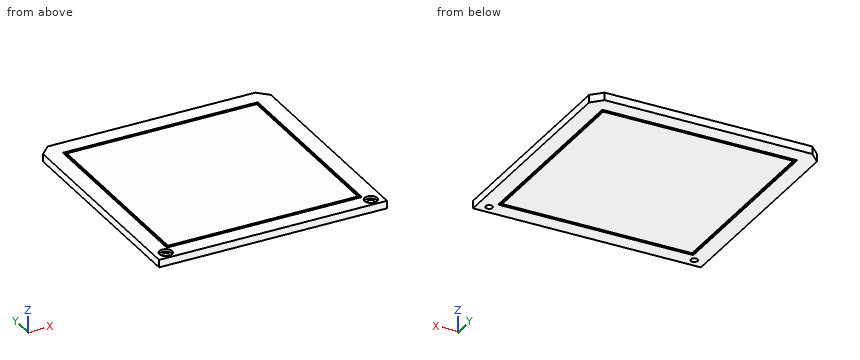
```python
from build123d import *

# Parameters (mm, degrees)
SKETCH1_W           = 90
SKETCH1_H           = 90
BOSS_EXTRUDE1_DEPTH = 3
SKETCH2_R           = 1.35
CUT_EXTRUDE1_DEPTH  = 4
SKETCH3_W           = 77
SKETCH3_H           = 77
SKETCH3_W_2         = 75
SKETCH3_H_2         = 75
CUT_EXTRUDE2_DEPTH  = 0.4
SKETCH4_W           = 77
SKETCH4_H           = 77
SKETCH4_W_2         = 75
SKETCH4_H_2         = 75
CUT_EXTRUDE3_DEPTH  = 0.4
CHAMFER1_SIZE       = 4
SKETCH5_R           = 2.5
CUT_EXTRUDE4_DEPTH  = 1


with BuildPart() as part:
    # Sketch1 → Boss-Extrude1 (new body)
    with BuildSketch(Plane.XY):
        Rectangle(SKETCH1_W, SKETCH1_H)
    extrude(amount=BOSS_EXTRUDE1_DEPTH)

    # Sketch2 → Cut-Extrude1 (cut, through all)
    with BuildSketch(Plane.XY.offset(3)):
        with Locations((-40.5, -41.5)):
            Circle(SKETCH2_R)
        with Locations((40.5, -41.5)):
            Circle(SKETCH2_R)
    extrude(amount=-CUT_EXTRUDE1_DEPTH, mode=Mode.SUBTRACT)

    # Sketch3 → Cut-Extrude2 (cut)
    with BuildSketch(Plane.XY.offset(3)):
        Rectangle(SKETCH3_W, SKETCH3_H)
        Rectangle(SKETCH3_W_2, SKETCH3_H_2, mode=Mode.SUBTRACT)
    extrude(amount=-CUT_EXTRUDE2_DEPTH, mode=Mode.SUBTRACT)

    # Sketch4 → Cut-Extrude3 (cut)
    with BuildSketch(Plane(origin=(0, 0, 0), x_dir=(-1, 0, 0), z_dir=(0, 0, -1))):
        Rectangle(SKETCH4_W, SKETCH4_H)
        Rectangle(SKETCH4_W_2, SKETCH4_H_2, mode=Mode.SUBTRACT)
    extrude(amount=-CUT_EXTRUDE3_DEPTH, mode=Mode.SUBTRACT)

    # Chamfer1
    chamfer1_edges = [part.edges().sort_by_distance(p)[0] for p in [
        (-45, 45, 1.5),
        (45, 45, 1.5),
    ]]
    chamfer(chamfer1_edges, length=CHAMFER1_SIZE)

    # Sketch5 → Cut-Extrude4 (cut)
    with BuildSketch(Plane.XY.offset(3)):
        with Locations((-40.5, -41.5)):
            Circle(SKETCH5_R)
        with Locations((40.5, -41.5)):
            Circle(SKETCH5_R)
    extrude(amount=-CUT_EXTRUDE4_DEPTH, mode=Mode.SUBTRACT)


solid = part.part
```
Work out the finished part from the listing and answer in its coordinate system (mm). Give positions to 0.01 mm unless a question says otherwise; leave off trailing zeros. Loops run counter-clockwise (first coordinate to the right, second up) from the corner with the lowest first, then second, coordinate; pieces in that order, holes last. Notation, with made-up numbers: (6.25, -16) - (28.25, -16) arc R6 ccw to (28.25, -6) - close; hole circle Ø1 at (8, 39.25). An arc over 180 degrees is marked (long way). Use CSV: the item, a comma, the result in double quotes. Start each with the question number.
(1) Find the intervals of material crossed by L1, parallel to X at y = 15.5, z = 2.9; L2, parallel to Y at x = 40.5, z = 1.4; L3, parallel to Y at x = -39.5, z = 1.2, in increasing order.
(2) This flat-tipped pin is pushed along its axis until it touches: pin 1 (8 mm diameter, centred on x = 26.5, y = 33.5, fed in from -Z). Where does it stop, or does it pass through?
(3) Find section A-A, the plane y = -41.5. Determine the outline of the cut face in (x, z), plus the area to 3 significant figures.
Results found:
1,L1,"-45 to -38.5, -37.5 to 37.5, 38.5 to 45"
1,L2,"-45 to -42.85, -40.15 to 45"
1,L3,"-45 to -42.41, -40.59 to 45"
2,pin 1,"z = 0"
3,outline,"(-45, 0) - (-41.85, 0) - (-41.85, 2) - (-43, 2) - (-43, 3) - (-45, 3) - close; (-39.15, 0) - (39.15, 0) - (39.15, 2) - (38, 2) - (38, 3) - (-38, 3) - (-38, 2) - (-39.15, 2) - close; (41.85, 0) - (45, 0) - (45, 3) - (43, 3) - (43, 2) - (41.85, 2) - close"
3,area,"249 mm^2"
